The model under review builds one solid part; all positions refer to its coordinate system, in mm. Round coordinates to 2 decimals unless told otherwise and drop trailing zeros. Order: outer loops, then holes, each group sorted by start corner. A loop starts at its lowest first (then second) coordinate and runs counter-clockwise, first axis right, second up.
1) To check wall thickness, follow L1, parallel to Z at x = 5, y = -25.4; L2, parallel to Y at x = 3.5, z = -25.4 (3 decimals); L3, parallel to Y at x = 4.25, z = -23.5 (3 decimals). State the ranges of each line that lie inside material, in increasing order.
2) Consider section C-C (x = 0.75). Give the boundary of the cut face in (y, z) (3 decimals), then the cut area to 3 significant figures.
3) Consider section A-A (z = -25.4). Give the boundary of the cut face in (x, y) (3 decimals), then the cut area to 3 significant figures.
4) Mouldability with a two-part tool opening along Z and no side actions: class faces 1 (the face through (3, -20.955, -25)), 2 (the face through (0, -39, -25)), 3 (the face through (3, -38, 0)), 4 (the face through (3.219, -31.747, -25.191)) as pulls with the +Z half, pulls with the -Z half, needs draft (parallel to the pull), parting line crosses it, or undercut.
5) Consider section B-B (y = -25.4). Give the boundary of the cut face in (x, z), then the cut area to 3 significant figures.
Autodesk Inventor part; units mm, degrees
ref_plane "YZ Plane" through (0, 0, 0) normal (1, 0, 0) x (0, 1, 0)
ref_plane "XZ Plane" through (0, 0, 0) normal (0, 1, 0) x (-1, 0, 0)
ref_plane "XY Plane" through (0, 0, 0) normal (0, 0, 1) x (1, 0, 0)
sketch "Sketch1" plane through (0, 0, 0) normal (1, 0, 0) x (0, 1, 0)
  line L0 (0, 0) -> (-76.2, 0)
  line L1 (-76.2, 0) -> (-76.2, -50.8)
  line L2 (-76.2, -50.8) -> (0, -50.8)
  line L3 (0, -50.8) -> (0, 0)
  dimension "d0" = 76.2
  dimension "d1" = 50.8
extrude "Extrusion1" add sketch "Sketch1" along normal blind 6.35
sketch "Sketch2" plane through (0, 0, 0) normal (-1, 0, 0) x (0, 0, 1)
  line L0 (-50.8, -76.2) -> (-50.8, 0)
  line L1 (0, 0) -> (0, -76.2)
  line L2 (-50.8, 0) -> (0, 0)
  point P0 (-25.4, -25.4)
  dimension "d4" = 50.8
  dimension "d5" = 25.4
  dimension "d6" = 25.4
hole "Hole1" at (0, -25.4, -25.4) direction (1, 0, 0) diameter 12.7 depth 25.4 tip angle 118
sketch "Sketch3" plane through (0, 0, 0) normal (-1, 0, 0) x (0, 0, 1)
  circle A0 centre (-25.4, -25.4) radius 6.35
  line L0 (0, 0) -> (0, -76.2)
  line L1 (-50.8, 0) -> (0, 0)
  line L2 (-50.8, -76.2) -> (-50.8, 0)
  line L3 (0, -76.2) -> (-50.8, -76.2)
  circle A1 centre (-25.4, -25.4) radius 6.35
  line L4 (-29.9348, -20.955) -> (-20.8652, -20.955)
  line L5 (-50.8, 0) -> (0, 0)
  dimension "d14" = 4.445
extrude "Extrusion2" add sketch "Sketch3" against normal blind 6.35 contours L4 A0 picked at (-25.16, -20.3336)
properties part number "StressTestPlate"
Answer below:
1. L1: z = -50.8 to -31.75, -19.05 to 0
1. L2: y = -76.2 to -31.75, -20.955 to 0
1. L3: y = -76.2 to -31.459, -20.955 to 0
2. outline: (-76.2, -50.8) - (0, -50.8) - (0, 0) - (-76.2, 0) - close; hole (-20.955, -29.935) - (-20.955, -20.865) arc R6.35 ccw (long way) to start
2. area: 3,760 mm2
3. outline: (0, -76.2) - (6.35, -76.2) - (6.35, -31.75) - (0, -31.75) - close; (0, -20.955) - (6.35, -20.955) - (6.35, 0) - (0, 0) - close
3. area: 415 mm2
4. face 1: undercut
4. face 2: needs draft
4. face 3: pulls with the +Z half
4. face 4: undercut
5. outline: (0, -50.8) - (6.35, -50.8) - (6.35, -31.75) - (0, -31.75) - close; (0, -19.05) - (6.35, -19.05) - (6.35, 0) - (0, 0) - close
5. area: 242 mm2
